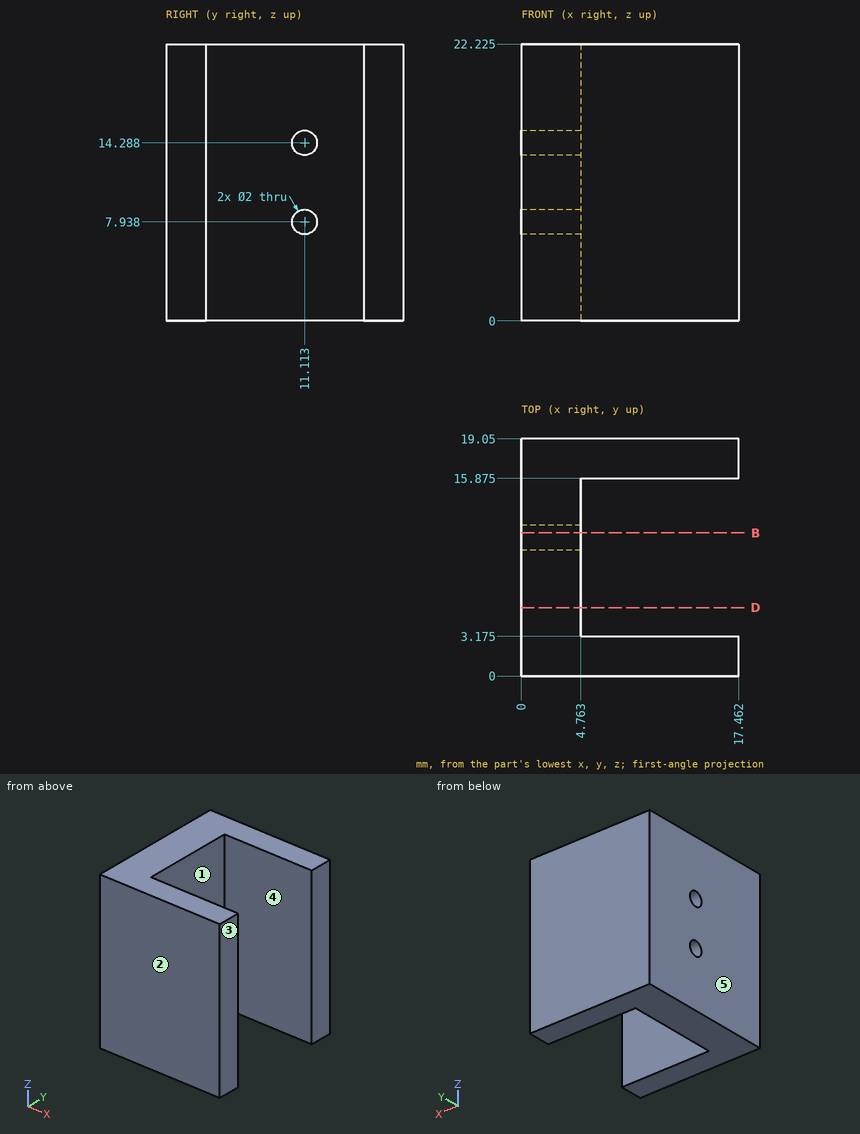
Geometry check sheet. Reference: drawing and pictorial views, mm from the part's lowest x, y, z. A direction names the side the tool comes from. Give positions to 0.01 mm unless a question says otherwise; leave off trailing zeros. Write each loop counter-clockwise with the first axis right and the second up, starting at its lowest first coordinate (ties: lowest second). Pieces come first, ordered by that corner, then holes. Notation, with made-up numbers: (11, 69) - (34, 69) arc R19 ccw to (34, 75) - close; hole circle Ø2 at (26.25, 32.5). An arc over 180 degrees is marked (long way). Use a Markdown table: item, result.
Q1. Go/stop test with a flat-tipped pin: P1, Ø2.5, axis at y = 11.11, z = 7.94, coming from the +X side. Record where the tip stops, or that it passes through.
Computed:
| item | result |
|---|---|
| P1 | stops at x = 4.76 |
Q2. Set-up check for the marked faces 4 and 5: record each of +Z, -Z, +X, -X, +Y, -Y from which the full face is reachable in a straight line by a thin tool's end or side.
Computed:
| item | result |
|---|---|
| face 4 | +Z, -Z, +X |
| face 5 | +Z, -Z, -X, +Y, -Y |
Q3. Draft check along Y on the marked faces 1, 2 and 3. Enter one of: pulls with the +Y half, pulls with the -Y half, needs draft (parallel to the pull), parting line crosses it, or undercut.
Computed:
| item | result |
|---|---|
| face 1 | undercut |
| face 2 | pulls with the -Y half |
| face 3 | needs draft |
Q4. Thickness scan on L1, parallel to Z at x = 1.25, y = 10.5 (1 decimal); L2, parallel to X at y = 10, z = 11.75. Record the ranges inside material, lowest first. Write a range as [from, to].
Computed:
| item | result |
|---|---|
| L1 | z = [0, 7.1], [8.7, 13.5], [15.1, 22.2] |
| L2 | x = [0, 4.76] |
Q5. Section check D-D, the plane y = 5.5. Enter the section's corners in (x, z) (1 decimal), then the cut area to 3 significant figures.
Computed:
| item | result |
|---|---|
| outline | (0, 0) - (4.8, 0) - (4.8, 22.2) - (0, 22.2) - close |
| area | 106 mm² |
Q6. Section check B-B, the plane y = 11.5. Enter the section's corners in (x, z) (1 decimal).
Computed:
| item | result |
|---|---|
| outline | (0, 0) - (4.8, 0) - (4.8, 7) - (0, 7) - close; (0, 8.9) - (4.8, 8.9) - (4.8, 13.4) - (0, 13.4) - close; (0, 15.2) - (4.8, 15.2) - (4.8, 22.2) - (0, 22.2) - close |
